For this review, use the dimensioned drawing (mm, ordinates from the lowest corner) and the shaded views. Round coordinates to 2 decimals unless told otherwise and drop trailing zeros. Write each loop counter-clockwise with the first axis right and the second up, starting at its lowest first coordinate (ties: lowest second). Pieces come first, ordered by that corner, then holes. Notation, with made-up numbers: M 2.5,54 L 30.5,54 A19 cw 30.5,66 Z; hole C -25,-20.75 d4. An arc over 180 degrees is marked long. Use CSV: the item, a comma, the result in double quotes.
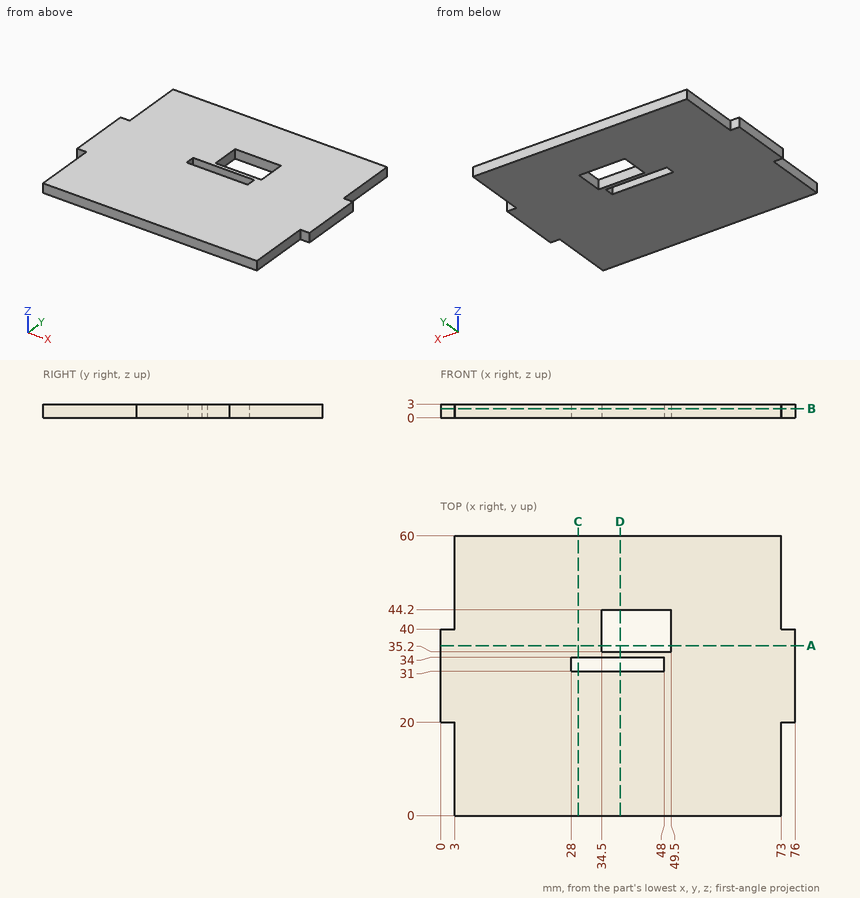
1) For pin 1 Ø0.9 at (y, z) = (11.5, 1) entering from +X; pin 2 Ø1.5 at (y, z) = (12.5, 2.5) entering from -X; pin 3 Ø0.9 at (x, z) = (75, 1.5) entering from -Y, all flat-tipped, find the tip position at first contact; note any pin that passes through.
Answers:
pin 1,"x = 73"
pin 2,"x = 3"
pin 3,"y = 20"
2) Add section D-D on x = 38.5. Write out the cut boundary in (y, z).
Answers:
outline,"M 0,0 L 31,0 L 31,3 L 0,3 Z; M 34,0 L 35.2,0 L 35.2,3 L 34,3 Z; M 44.2,0 L 60,0 L 60,3 L 44.2,3 Z"
3) Add section B-B on z = 2. Write out the cut boundary in (x, y), then the cut area to 4 significant figures.
Answers:
outline,"M 0,20 L 3,20 L 3,0 L 73,0 L 73,20 L 76,20 L 76,40 L 73,40 L 73,60 L 3,60 L 3,40 L 0,40 Z; hole M 28,31 L 48,31 L 48,34 L 28,34 Z; hole M 34.5,35.2 L 49.5,35.2 L 49.5,44.2 L 34.5,44.2 Z"
area,"4,125 mm²"
4) Add section C-C on x = 29.5. Write out the cut boundary in (y, z).
Answers:
outline,"M 0,0 L 31,0 L 31,3 L 0,3 Z; M 34,0 L 60,0 L 60,3 L 34,3 Z"
5) Wall thickness on line 1 along Y through (x, z) = (46, 2.25); line 2 along X through (y, z) = (38, 2); line 3 along X through (y, z) = (32.5, 1.25): over which ranges is each line inside the solid? List them lowest first. Write a range as [from, to].
Answers:
line 1,"[0, 31], [34, 35.2], [44.2, 60]"
line 2,"[0, 34.5], [49.5, 76]"
line 3,"[0, 28], [48, 76]"
6) Add section A-A on y = 36.5. Write out the cut boundary in (x, z).
Answers:
outline,"M 0,0 L 34.5,0 L 34.5,3 L 0,3 Z; M 49.5,0 L 76,0 L 76,3 L 49.5,3 Z"
